```python
from build123d import *

# Parameters (mm, degrees)
SALIENTE_EXTRUIR1_DEPTH = 6
CROQUIS2_R              = 1.7
CORTAR_EXTRUIR1_DEPTH   = 7
CROQUIS3_R              = 3.4
CROQUIS3_R_2            = 1.7
SALIENTE_EXTRUIR2_DEPTH = 6


with BuildPart() as part:
    # Croquis1 → Saliente-Extruir1 (new body)
    with BuildSketch(Plane.XY):
        with BuildLine():
            Line((-45.5, 0), (-35.5, 0))
            ThreePointArc((-35.5, 0), (0, 35.5), (35.5, 0))
            Line((35.5, 0), (45.5, 0))
            ThreePointArc((45.5, 0), (0, 45.5), (-45.5, 0))
        make_face()
    extrude(amount=SALIENTE_EXTRUIR1_DEPTH)

    # Croquis2 → Cortar-Extruir1 (cut, through all)
    with BuildSketch(Plane.XY.offset(6)):
        with Locations((0, 40.5)):
            Circle(CROQUIS2_R)
        with Locations((28.637824638, 28.637824638)):
            Circle(CROQUIS2_R)
        with Locations((40.5, 0)):
            Circle(CROQUIS2_R)
        with Locations((-40.5, 0)):
            Circle(CROQUIS2_R)
        with Locations((-28.637824638, 28.637824638)):
            Circle(CROQUIS2_R)
    extrude(amount=-CORTAR_EXTRUIR1_DEPTH, mode=Mode.SUBTRACT)

    # Croquis3 → Saliente-Extruir2 (add)
    with BuildSketch(Plane.XY.offset(6)):
        with Locations((-40.5, 0)):
            Circle(CROQUIS3_R)
        with Locations((-40.5, 0)):
            Circle(CROQUIS3_R_2, mode=Mode.SUBTRACT)
        with Locations((40.5, 0)):
            Circle(CROQUIS3_R)
        with Locations((40.5, 0)):
            Circle(CROQUIS3_R_2, mode=Mode.SUBTRACT)
    extrude(amount=-SALIENTE_EXTRUIR2_DEPTH)


solid = part.part
```
Build history of the part. All positions in model axes, mm. A direction names the side the tool comes from. Round coordinates to 2 decimals unless told otherwise and drop trailing zeros. Write each loop counter-clockwise with the first axis right and the second up, starting at its lowest first coordinate (ties: lowest second). Pieces come first, ordered by that corner, then holes. Notation, with made-up numbers: (-29, 41.5) - (0, 41.5) arc R25 ccw to (0, 63.5) - close; hole circle Ø10 at (8.5, -35.5). An arc over 180 degrees is marked (long way). Write each question's results on one line, items separated by ' | '. Start each with the question number.
Item 1: Saw through at D-D (x = 25.5). Write the cut outline in (y, z), and give its area (3 significant figures).
Item 2: Drop flat-ended pins along their axis: P1, Ø1.5, axis at y = 36.5, z = 2, coming from the +X side; P2, Ø2, axis at y = 27, z = 3.5, coming from the +X side; P3, Ø0.8, axis at x = 44.5, z = 2, coming from the -Y side. Give the stop position or say it passes through.
Item 3: Saw through at A-A (x = 0). Write the cut outline in (y, z).
Item 4: Saw through at C-C (z = 3.55). Write the cut outline in (x, y).
Item 5: Which spindle directions (+Z, -Z, +X, -X, +Y, -Y) get a long thin tool onto all of the face, cutting with end or side? Do faces 1 (the face through (29.42, 27.13, 3.04)), 2 (the face through (36, 0, 3)), 3 (the face through (45, 0, 3)), 4 (the face through (-45, 0, 3)). Say none if no direction does.
Item 6: Mould opens along Y. For faces 5 (the face through (-27.85, 27.13, 3.04)), 6 (the face through (-0.78, 35.49, 2.96)), 7 (the face through (1, 45.49, 2.96)) say: pulls with the +Y half, pulls with the -Y half, needs draft (parallel to the pull), parting line crosses it, or undercut.
Item 7: Wall check: L1, parallel to Y at x = 0, z = 4.05; L2, parallel to X at y = 29, z = 2.7; L3, parallel to X at y = 11.5, z = 3.55. Give the ranges that are in metal, low to high. Write a range as [from, to].
Item 8: Saw through at B-B (y = 22). Write the cut outline in (x, z), and give its area (3 significant figures).
Results are:
1) outline: (24.7, 0) - (37.68, 0) - (37.68, 6) - (24.7, 6) - close | area: 77.9 mm²
2) P1: stops at x = 28.15 | P2: stops at x = 37.34 | P3: stops at y = 0
3) outline: (35.5, 0) - (38.8, 0) - (38.8, 6) - (35.5, 6) - close; (42.2, 0) - (45.5, 0) - (45.5, 6) - (42.2, 6) - close
4) outline: (-45.5, 0) - (-43.9, 0) arc R3.4 ccw to (-37.1, 0) - (-35.5, 0) arc R35.5 cw to (35.5, 0) - (37.1, 0) arc R3.4 ccw to (43.9, 0) - (45.5, 0) arc R45.5 ccw to start; hole circle Ø3.4 at (-40.5, 0); hole circle Ø3.4 at (-28.64, 28.64); hole circle Ø3.4 at (0, 40.5); hole circle Ø3.4 at (28.64, 28.64); hole circle Ø3.4 at (40.5, 0)
5) face 1: +Z, -Z | face 2: +Z, -Z, -Y | face 3: +Z, -Z, +X, -Y | face 4: +Z, -Z, -X, -Y
6) face 5: undercut | face 6: pulls with the -Y half | face 7: pulls with the +Y half
7) L1: y = [35.5, 38.8], [42.2, 45.5] | L2: x = [-35.06, -30.3], [-26.98, -20.48], [20.48, 26.98], [30.3, 35.06] | L3: x = [-44.02, -33.59], [33.59, 44.02]
8) outline: (-39.83, 0) - (-27.86, 0) - (-27.86, 6) - (-39.83, 6) - close; (27.86, 0) - (39.83, 0) - (39.83, 6) - (27.86, 6) - close | area: 144 mm²
